Geometry: final body of the model. Coordinates: model frame, mm. A direction names the side the tool comes from. Give positions to 0.01 mm unless a question says otherwise; leave off trailing zeros. Write each loop counter-clockwise with the first axis right and the second up, starting at its lowest first coordinate (ties: lowest second). Pieces come first, ordered by that corner, then holes. Notation, with made-up numbers: (-12, -24) -> (4, -24) arc R18 cw to (4, -9) -> close; hole circle Ø1 at (7.25, 35.25). An arc over 180 degrees is marked (long way). Answer as a JSON object with one key per item and string values.
from build123d import *

# Parameters (mm, degrees)
SKETCH_1_R          = 12.5
EXTRUDE_1_DEPTH     = 56
SKETCH_4_R          = 7
EXTRUDE_2_DEPTH     = 3
SKETCH_7_R          = 7
EXTRUDE_3_DEPTH     = 20
CHAMFER_1_SIZE      = 2
SKETCH_8_R          = 7
CUT_EXTRUDE_3_DEPTH = 33.5
SKETCH_9_R          = 14.5
SKETCH_9_R_2        = 12.5
EXTRUDE_4_DEPTH     = 7
SKETCH_10_R         = 2.75
CUT_EXTRUDE_4_DEPTH = 79.71785058
CUT_EXTRUDE_5_DEPTH = 2.5
SKETCH_12_W         = 5
SKETCH_12_H         = 4.425702811
CUT_EXTRUDE_6_DEPTH = 30
CHAMFER_2_SIZE      = 0.5
CHAMFER_3_SIZE      = 0.5
CHAMFER_4_SIZE      = 0.5
CHAMFER_5_SIZE      = 0.5
FILLET_1_R          = 1


with BuildPart() as part:
    # 草图1 → 拉伸1 (new body)
    with BuildSketch(Plane.XY):
        Circle(SKETCH_1_R)
    extrude(amount=EXTRUDE_1_DEPTH)

    # 草图4 → 拉伸2 (add)
    with BuildSketch(Plane.XY.offset(56)):
        Circle(SKETCH_4_R)
    extrude(amount=-EXTRUDE_2_DEPTH)

    # 草图7 → 拉伸3 (add)
    with BuildSketch(Plane.XY.offset(56)):
        Circle(SKETCH_7_R)
    extrude(amount=EXTRUDE_3_DEPTH)

    # 倒角1
    chamfer_1_edges = [part.edges().sort_by_distance(p)[0] for p in [
        (-12.5, 0, 56),
    ]]
    chamfer(chamfer_1_edges, length=CHAMFER_1_SIZE)

    # 草图8 → 切除-拉伸3 (cut)
    with BuildSketch(Plane(origin=(0, 0, 0), x_dir=(-1, 0, 0), z_dir=(0, 0, -1))):
        with Locations(Location((0, 0, 0), (0, 0, 180))):
            Circle(SKETCH_8_R)
    extrude(amount=-CUT_EXTRUDE_3_DEPTH, mode=Mode.SUBTRACT)

    # 草图9 → 拉伸4 (add)
    with BuildSketch(Plane(origin=(0, 0, 0), x_dir=(-1, 0, 0), z_dir=(0, 0, -1))):
        Circle(SKETCH_9_R)
        Circle(SKETCH_9_R_2, mode=Mode.SUBTRACT)
    extrude(amount=-EXTRUDE_4_DEPTH)

    # 草图10 → 切除-拉伸4 (cut, through all)
    with BuildSketch(Plane.XY.offset(76)):
        Circle(SKETCH_10_R)
    extrude(amount=-CUT_EXTRUDE_4_DEPTH, mode=Mode.SUBTRACT)

    # 草图11 → 切除-拉伸5 (cut)
    with BuildSketch(Plane(origin=(0, 7, 0), x_dir=(-1, 0, 0), z_dir=(0, 1, 0))):
        with BuildLine():
            Line((-2.5, 73), (-2.5, 58.5))
            ThreePointArc((-2.5, 58.5), (0, 56), (2.5, 58.5))
            Line((2.5, 58.5), (2.5, 73))
            ThreePointArc((2.5, 73), (0, 75.5), (-2.5, 73))
        make_face()
    extrude(amount=-CUT_EXTRUDE_5_DEPTH, mode=Mode.SUBTRACT)

    # 草图12 → 切除-拉伸6 (cut)
    with BuildSketch(Plane(origin=(0, 0, 0), x_dir=(-1, 0, 0), z_dir=(0, 0, -1))):
        with Locations((0, 6.787148594)):
            Rectangle(SKETCH_12_W, SKETCH_12_H)
    extrude(amount=-CUT_EXTRUDE_6_DEPTH, mode=Mode.SUBTRACT)

    # 倒角2
    chamfer_2_edges = [part.edges().sort_by_distance(p)[0] for p in [
        (14.5, 0, 7),
        (14.5, 0, 0),
        (-3.968626967, -5.766281297, 0),
    ]]
    chamfer(chamfer_2_edges, length=CHAMFER_2_SIZE)

    # 倒角3
    chamfer_3_edges = [part.edges().sort_by_distance(p)[0] for p in [
        (-7, 0, 76),
    ]]
    chamfer(chamfer_3_edges, length=CHAMFER_3_SIZE - 0.0001)  # a hair under: the kernel refuses the full size

    # 倒角4
    chamfer_4_edges = [part.edges().sort_by_distance(p)[0] for p in [
        (-2.75, 0, 76),
    ]]
    chamfer(chamfer_4_edges, length=CHAMFER_4_SIZE)

    # 倒角5
    chamfer_5_edges = [part.edges().sort_by_distance(p)[0] for p in [
        (-2.75, 0, 33.5),
    ]]
    chamfer(chamfer_5_edges, length=CHAMFER_5_SIZE)

    # 圆角1
    fillet_1_edges = [part.edges().sort_by_distance(p)[0] for p in [
        (-7, 0, 33.5),
    ]]
    fillet(fillet_1_edges, radius=FILLET_1_R)


solid = part.part
Q1. Cut plane B-B (z = 47). Return the cut outline in (x, y).
Values:
{"outline": "circle Ø25 at (0, 0); hole circle Ø5.5 at (0, 0)"}
Q2. Set-up query: faces 1 (the flat face through (-2.5, 8, 15)), 2 (the flat face through (-6, -6, 0)), 3 (the flat face through (2.5, 6, 66)). Return all of +Z, -Z, +X, -X, +Y, -Y with unobstructed straight access to the full face (end or side cutting, diameter ignored); none if empty.
Values:
{"face 1": "-Z", "face 2": "-Z, +X, -X, +Y, -Y", "face 3": "+Y"}
Q3. Mould query, pull axis Z, two halves, no side actions, for faces 4 (the flat face through (5.3, 11.5, 7)), 5 (the cylindrical face through (11.923, 3.755, 30.171)), 6 (the cylindrical face through (0, 6, 56)). Classes: pulls with the +Z half, pulls with the -Z half, needs draft (parallel to the pull), parting line crosses it, or undercut.
Values:
{"face 4": "pulls with the +Z half", "face 5": "needs draft", "face 6": "undercut"}
Q4. Material intervals for L1, parallel to Y at x = 0, z = 25; L2, parallel to Z at x = 6, y = -11.5; L3, parallel to Y at x = 0, z = 61, sorted ascending. Write a range as from..to.
Values:
{"L1": "-12.5..-7, 9..12.5", "L2": "0..7", "L3": "-7..-2.75, 2.75..4.5"}
Q5. First-contact query: P1, Ø2, axis at y = 5, z = 65, coming from the +X side; P2, Ø1.2, axis at y = 8.5, z = 20, coming from the +X side; P3, Ø0.7, axis at y = 8.5, z = 11.5, coming from the -X side. Flat tips, straight axial feed; report the tip coordinate or a pass-through.
Values:
{"P1": "x = 5.74", "P2": "x = 9.69", "P3": "x = -9.48"}
Q6. Cut plane A-A (z = 25). Return the cut outline in (x, y).
Values:
{"outline": "circle Ø25 at (0, 0); hole (-2.5, 6.54) arc R7 ccw (long way) to (2.5, 6.54) -> (2.5, 9) -> (-2.5, 9) -> close"}
